Can you work these out from the model? Positions are in its coordinate system, mm. Round coordinates to 2 decimals unless told otherwise and drop trailing zeros. Order: outer loops, then holes, each group sorted by start corner. A loop starts at its lowest first (then second) coordinate and runs counter-clockwise, first axis right, second up. Notation, with made-up numbers: (18.25, 56) -> (67.25, 56) arc R19 cw to (67.25, 87) -> close; hole circle Ø9 at (53, -26). An arc over 180 degrees is marked (long way). Use a Markdown table: item, result. Add a question column.
Q1. If we section it at A-A on y = 0: List the corners of the cut face in (x, z) for me (3 decimals), plus the area to 3 significant figures.
Q2. I need wall thicknesses on line 1 along Y through (x, z) = (0, 0.4) (3 decimals); line 2 along X through (y, z) = (-25, 0.75). Which ranges of each line are inside material? Lowest first, please. Write a range as [from, to].
Q3. If we section it at C-C on z = 1.8: Give the number of separate pieces and of enclosed holes in the cut face, plus the area to 3 significant figures.
Q4. I'm going to push flat-ended pins straight in: pin 1 Ø23 at (x, y) = (0, 0) entering from +Z; pin 2 Ø1 at (x, z) = (-12.5, 2) entering from -Y; pin 3 Ø1.6 at (x, y) = (24, 0) entering from +Z; pin 4 Ø1 at (y, z) = (-9, 2.5) entering from -X. Where does each tip first touch, or does it pass through?
Q5. If we section it at D-D on x = -14.5: List the corners of the cut face in (y, z) for me.
```python
from build123d import *

# Parameters (mm, degrees)
SKETCH1_R           = 1.4
BOSS_EXTRUDE1_DEPTH = 3
CUT_EXTRUDE1_DEPTH  = 2
CUT_EXTRUDE2_REACH  = 47.001
SKETCH3_R           = 8.775


with BuildPart() as part:
    # Sketch1 → Boss-Extrude1 (new body)
    with BuildSketch(Plane.XY):
        with BuildLine():
            ThreePointArc((6.75, 25), (0, 31.75), (-6.75, 25))
            ThreePointArc((-6.75, 25), (-8.128131702, 18.306346632), (-12.038357667, 12.701493797))
            ThreePointArc((-12.038357667, 12.701493797), (-12.374368671, 12.374368671), (-12.701493797, 12.038357667))
            ThreePointArc((-12.701493797, 12.038357667), (-18.306346632, 8.128131702), (-25, 6.75))
            ThreePointArc((-25, 6.75), (-31.75, 0), (-25, -6.75))
            ThreePointArc((-25, -6.75), (-18.306346632, -8.128131702), (-12.701493797, -12.038357667))
            ThreePointArc((-12.701493797, -12.038357667), (-12.374368671, -12.374368671), (-12.038357667, -12.701493797))
            ThreePointArc((-12.038357667, -12.701493797), (-8.128131702, -18.306346632), (-6.75, -25))
            ThreePointArc((-6.75, -25), (0, -31.75), (6.75, -25))
            ThreePointArc((6.75, -25), (8.128131702, -18.306346632), (12.038357667, -12.701493797))
            ThreePointArc((12.038357667, -12.701493797), (12.374368671, -12.374368671), (12.701493797, -12.038357667))
            ThreePointArc((12.701493797, -12.038357667), (18.306346632, -8.128131702), (25, -6.75))
            ThreePointArc((25, -6.75), (31.75, 0), (25, 6.75))
            ThreePointArc((25, 6.75), (18.306346632, 8.128131702), (12.701493797, 12.038357667))
            ThreePointArc((12.701493797, 12.038357667), (12.374368671, 12.374368671), (12.038357667, 12.701493797))
            ThreePointArc((12.038357667, 12.701493797), (8.128131702, 18.306346632), (6.75, 25))
        make_face()
        with Locations((0, 25)):
            Circle(SKETCH1_R, mode=Mode.SUBTRACT)
        with Locations((-25, 0)):
            Circle(SKETCH1_R, mode=Mode.SUBTRACT)
        with Locations((0, -25)):
            Circle(SKETCH1_R, mode=Mode.SUBTRACT)
        with Locations((25, 0)):
            Circle(SKETCH1_R, mode=Mode.SUBTRACT)
    extrude(amount=BOSS_EXTRUDE1_DEPTH)

    # Sketch2 → Cut-Extrude1 (cut)
    with BuildSketch(Plane.XY.offset(3)):
        Polygon((3.117691454, 25), (1.558845727, 27.7), (-1.558845727, 27.7), (-3.117691454, 25), (-1.558845727, 22.3), (1.558845727, 22.3), align=None)
        Polygon((25, 3.117691454), (22.3, 1.558845727), (22.3, -1.558845727), (25, -3.117691454), (27.7, -1.558845727), (27.7, 1.558845727), align=None)
        Polygon((3.117691454, -25), (1.558845727, -22.3), (-1.558845727, -22.3), (-3.117691454, -25), (-1.558845727, -27.7), (1.558845727, -27.7), align=None)
        Polygon((-25, -3.117691454), (-22.3, -1.558845727), (-22.3, 1.558845727), (-25, 3.117691454), (-27.7, 1.558845727), (-27.7, -1.558845727), align=None)
    extrude(amount=-CUT_EXTRUDE1_DEPTH, mode=Mode.SUBTRACT)

    # Sketch3 → Cut-Extrude2 (cut, up to next)
    with BuildSketch(Plane.XY.offset(3), mode=Mode.PRIVATE) as cut_extrude2_sk1:
        Circle(SKETCH3_R)
    cut_extrude2_tool1 = extrude(cut_extrude2_sk1.sketch, amount=-CUT_EXTRUDE2_REACH, mode=Mode.PRIVATE) & part.part
    add(cut_extrude2_tool1.solids().sort_by_distance((0, 0, 3))[0], mode=Mode.SUBTRACT)


solid = part.part
```
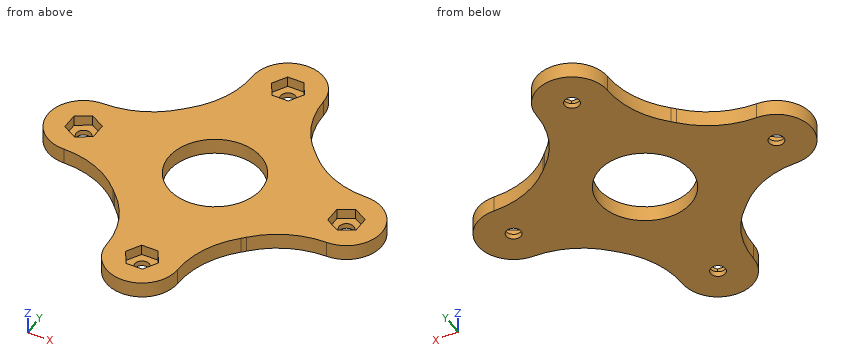
Answer below:
| question | item | result |
|---|---|---|
| 1 | outline | (-31.75, 0) -> (-26.4, 0) -> (-26.4, 1) -> (-27.7, 1) -> (-27.7, 3) -> (-31.75, 3) -> close; (-23.6, 0) -> (-8.775, 0) -> (-8.775, 3) -> (-22.3, 3) -> (-22.3, 1) -> (-23.6, 1) -> close; (8.775, 0) -> (23.6, 0) -> (23.6, 1) -> (22.3, 1) -> (22.3, 3) -> (8.775, 3) -> close; (26.4, 0) -> (31.75, 0) -> (31.75, 3) -> (27.7, 3) -> (27.7, 1) -> (26.4, 1) -> close |
| 1 | area | 111 mm² |
| 2 | line 1 | [-31.75, -26.4], [-23.6, -8.775], [8.775, 23.6], [26.4, 31.75] |
| 2 | line 2 | [-6.75, -1.4], [1.4, 6.75] |
| 3 | separate pieces | 1 |
| 3 | enclosed holes | 5 |
| 3 | area | 1,410 mm² |
| 4 | pin 1 | z = 3 |
| 4 | pin 2 | y = -12.74 |
| 4 | pin 3 | z = 1 |
| 4 | pin 4 | x = -17.5 |
| 5 | outline | (-10.4, 0) -> (10.4, 0) -> (10.4, 3) -> (-10.4, 3) -> close |
